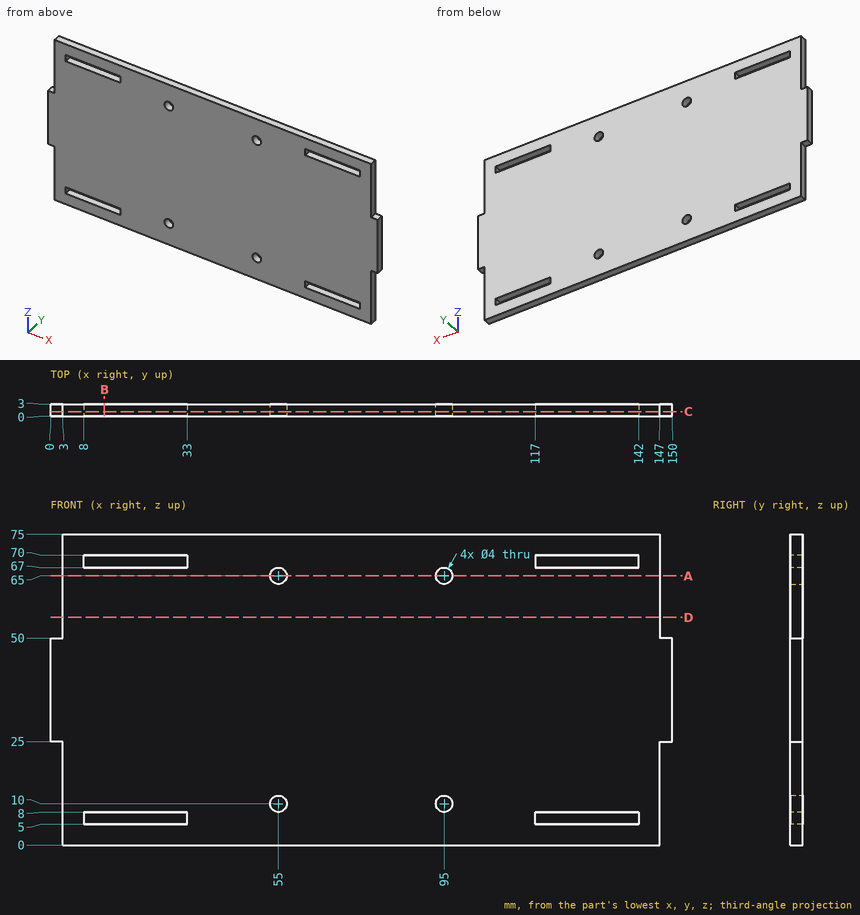
Here's the drawing with two shaded views (mm, measured from the low corner). I have some questions. Round coordinates to 2 decimals unless told otherwise and drop trailing zeros. Loops run counter-clockwise (first coordinate to the right, second up) from the corner with the lowest first, then second, coordinate; pieces in that order, holes last. Notation, with made-up numbers: (77, -37.5) -> (119, -37.5) arc R29 ccw to (119, 0.5) -> close; hole circle Ø7 at (49, 1). An arc over 180 degrees is marked (long way). Answer as CSV lines item,"result". Start each with the question number.
1. Imagine slicing it at B-B on x = 13. Write out the boundary of the cut face in (y, z), plus the area to 3 significant figures.
2. I need wall thicknesses on probe 1 along Z at (x, y) = (55, 1.6); probe 2 along Z at (x, y) = (27.5, 1.5); probe 3 along X at (y, z) = (1.9, 69.5). Which ranges of each line are inside material? Lowest first, please. Write a range as from..to.
3. Imagine slicing it at A-A on z = 65. Write out the boundary of the cut face in (x, y), plus the area to 3 significant figures.
4. I'm going to push flat-ended pins straight in: P1, Ø4, axis at x = 119, z = 34.5, coming from the -Y side; P2, Ø0.9, axis at y = 1, z = 69, coming from the +X side; P3, Ø0.9, axis at x = 149, y = 1.5, coming from the -Z side; P4, Ø0.9, axis at x = 148, y = 1, coming from the +Z side. Where does each tip first touch, or does it pass through?
5. Imagine slicing it at D-D on z = 55. Write out the boundary of the cut face in (x, y).
6. Imagine slicing it at C-C on y = 1.15. State how many separate pieces and enclosed holes the cut face has, plus the area to 3 significant figures.
Solution:
1,outline,"(0, 0) -> (3, 0) -> (3, 5) -> (0, 5) -> close; (0, 8) -> (3, 8) -> (3, 67) -> (0, 67) -> close; (0, 70) -> (3, 70) -> (3, 75) -> (0, 75) -> close"
1,area,"207 mm²"
2,probe 1,"0..8, 12..63, 67..75"
2,probe 2,"0..5, 8..67, 70..75"
2,probe 3,"3..8, 33..117, 142..147"
3,outline,"(3, 0) -> (53, 0) -> (53, 3) -> (3, 3) -> close; (57, 0) -> (93, 0) -> (93, 3) -> (57, 3) -> close; (97, 0) -> (147, 0) -> (147, 3) -> (97, 3) -> close"
3,area,"408 mm²"
4,P1,"y = 0"
4,P2,"x = 147"
4,P3,"z = 25"
4,P4,"z = 50"
5,outline,"(3, 0) -> (147, 0) -> (147, 3) -> (3, 3) -> close"
6,separate pieces,"1"
6,enclosed holes,"8"
6,area,"10,600 mm²"
